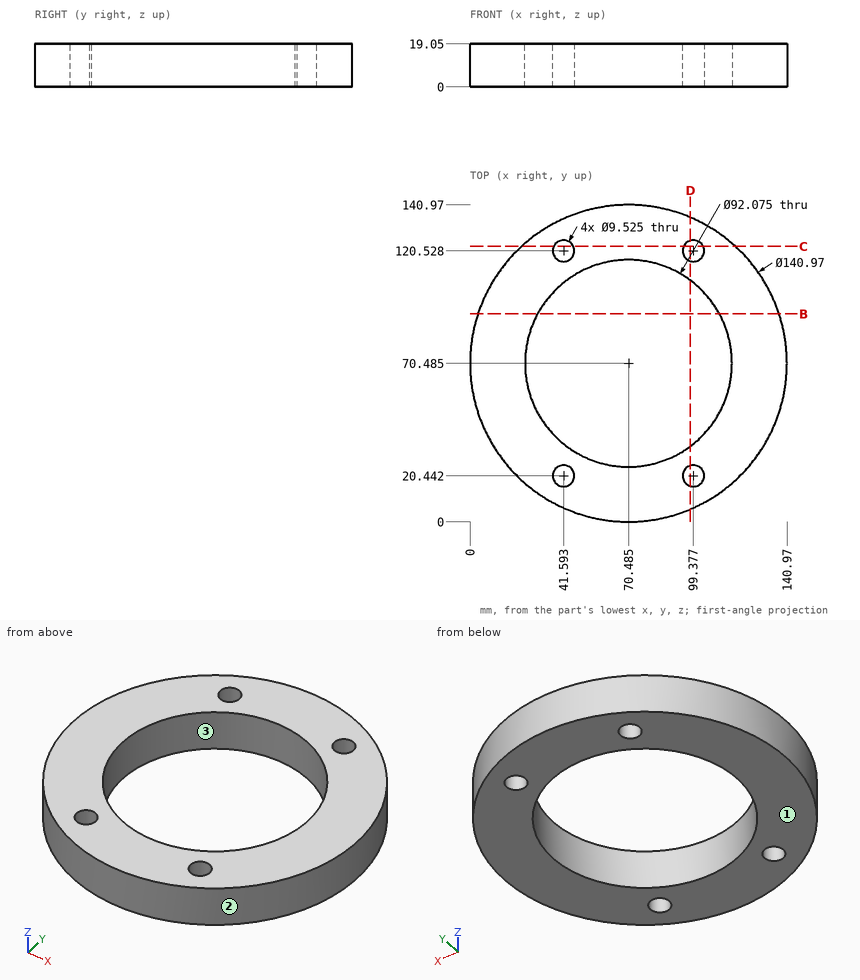
The figure shows three views and two pictorial views of one solid part (mm, origin at its lowest corner). Answer the questions. Coordinates: 2 decimals unless noted, no trailing zeros. Write each loop counter-clockwise with the first axis right and the second up, starting at its lowest first coordinate (ties: lowest second). Pieces come first, ordered by that corner, then holes.
1. The part is cut by section D-D, the plane x = 98. State how many separate pieces and enclosed holes the cut face has, and give its area (3 significant figures).
Results list:
separate pieces: 4
enclosed holes: 0
area: 719 mm2
2. The part is cut by section B-B, the plane y = 92.5. Write down the section's boundary in (x, z), and give its area (3 significant figures).
Results list:
outline: (3.53, 0) - (30.05, 0) - (30.05, 19.05) - (3.53, 19.05) - close; (110.92, 0) - (137.44, 0) - (137.44, 19.05) - (110.92, 19.05) - close
area: 1,010 mm2
3. For a pull along X with two mould halves and no side action, classify the marked faces 1, 2 and 3 as +X half, -X half, draft (parallel to the pull), parting line (faces both ways), or undercut.
Results list:
face 1: draft
face 2: parting line
face 3: undercut
4. Flat-ended cylindrical pins translate along their axes: pin 1 (1.5 mm diameter, centred on x = 107, z = 11.5, fed in from +Y); pin 2 (5 mm diameter, centred on x = 121, z = 7.5, fed in from +Y) (1 decimal); pin 3 (3 mm diameter, centred on x = 82.5, z = 5, fed in from +Y). Find the tip coordinate at first contact, or state that the pin passes through.
Results list:
pin 1: stops at y = 131.22
pin 2: stops at y = 122.1
pin 3: stops at y = 140.18
5. The part is cut by section C-C, the plane y = 122.5. Write down the section's boundary in (x, z).
Results list:
outline: (22.92, 0) - (37.26, 0) - (37.26, 19.05) - (22.92, 19.05) - close; (45.93, 0) - (95.04, 0) - (95.04, 19.05) - (45.93, 19.05) - close; (103.71, 0) - (118.05, 0) - (118.05, 19.05) - (103.71, 19.05) - close
6. Consider line 1 along X through (y, z) = (70.5, 9.5); line 2 along X through (y, z) = (18, 18) (1 decimal); line 3 along Y through (x, z) = (44.5, 18.25) (1 decimal). Determine where each line is inside the solid, lowest interval first.
Results list:
line 1: x = 0 to 24.45, 116.52 to 140.97
line 2: x = 23.4 to 37.5, 45.7 to 95.3, 103.5 to 117.5
line 3: y = 5 to 16.7, 24.2 to 32.5, 108.5 to 116.8, 124.3 to 136
